from build123d import *

# Parameters (mm, degrees)
SKETCH_R        = 2.25
SKETCH_W        = 6
SKETCH_H        = 28
PAD_DEPTH       = 4.1
POCKET_DEPTH    = 3.5
SKETCH003_W     = 21
SKETCH003_H     = 4.1
POCKET001_DEPTH = 1
SKETCH002_R     = 2.25
PAD001_DEPTH    = 0.3


with BuildPart() as part:
    # Sketch → Pad (new body)
    with BuildSketch(Plane.XY):
        Polygon((-10.5, 15.5), (10.5, 15.5), (10.5, 10.499836), (6, 5.999836), (6, -5.999836), (10.5, -10.499836), (10.5, -15.5), (-10.5, -15.5), (-10.5, -17.717136), (-10.5, -19.420319), (-13.45, -19.420319), (-19.053461, -16.18516), (-19.053461, -9.71484), (-13.45, -6.479681), (-10.500002, -6.479681), (-7.46388, -3.443559), (-7.46388, 7.463716), (-10.5, 10.499836), align=None)
        with Locations((-13.45, -12.95)):
            Circle(SKETCH_R, mode=Mode.SUBTRACT)
        with Locations((0, -0.5)):
            Rectangle(SKETCH_W, SKETCH_H, mode=Mode.SUBTRACT)
    extrude(amount=PAD_DEPTH)

    # Sketch001 → Pocket (cut)
    with BuildSketch(Plane.XY.offset(4.1)):
        Polygon((-13.45, -17.020319), (-9.925, -14.98516), (-9.925, -10.91484), (-13.45, -8.879681), (-16.975, -10.91484), (-16.975, -14.98516), align=None)
    extrude(amount=-POCKET_DEPTH, mode=Mode.SUBTRACT)

    # Sketch003 → Pocket001 (cut)
    with BuildSketch(Plane(origin=(0, 15.5, 0), x_dir=(-1, 0, 0), z_dir=(0, 1, 0))):
        with Locations((0, 2.05)):
            Rectangle(SKETCH003_W, SKETCH003_H)
    extrude(amount=-POCKET001_DEPTH, mode=Mode.SUBTRACT)

    # Sketch002 → Pad001 (new body)
    with BuildSketch(Plane.XY.offset(0.6)):
        with Locations((-13.45, -12.95)):
            Circle(SKETCH002_R)
    extrude(amount=-PAD001_DEPTH)


solid = part.part
Read the model definition and answer for the solid it produces. Units are mm, in the model's axes. A direction names the side the tool comes from. Round coordinates to 2 decimals unless told otherwise and drop trailing zeros. Loops run counter-clockwise (first coordinate to the right, second up) from the corner with the lowest first, then second, coordinate; pieces in that order, holes last.
Q1. Section A-A on y = -12.95 is taken. Write down the section's boundary in (x, z) (3 decimals), and give its area (3 significant figures).
Q2. Each of these flat-tipped pins is pushed along its axis until it touches: pin 1 (1.5 mm diameter, centred on x = -11.5, z = 2.5, fed in from +Y); pin 2 (1.2 mm diameter, centred on y = 5, z = 3, fed in from +X); pin 3 (3.5 mm diameter, centred on x = -13.45, y = -12.95, fed in from +Z). Where does it stop, or does it pass through?
Q3. Which of the six approach directions +Z, -Z, +X, -X, +Y, -Y give full straight-line access (tool end or side, diameter ignored) to faces 5 (the face through (-12, -6.48, 2)), 6 (the face through (-10.5, -17, 2)), 7 (the face through (-3, -1, 2)), 8 (the face through (-16.975, -13, 2)), 9 (the face through (8, 8, 2))?
Q4. Section B-B on z = 1.75 is taken. Write down the section's boundary in (x, y) (3 decimals).
Q5. Section D-D on y = 0.5 is taken. Write down the section's boundary in (x, z), and give its area (3 significant figures).
Q6. Determine the mould class of faces 1 (the face through (-16.213, -17.825, 2.021)), 2 (the face through (-15.237, -15.988, 2.374)), 3 (the face through (-11.663, -9.912, 2.374)), 4 (the face through (10.5, 13, 2)) for opening direction X: released by +X, released by -X, zero draft, split by the parting line, or undercut.
Q7. Section C-C on x = -6.75 is taken. Write down the section's boundary in (y, z), and give its area (3 significant figures).
Q8. Consider probe 1 along X at (y, z) = (-12.5, 3.25) (3 decimals); probe 2 along X at (y, z) = (-2, 2.95); probe 3 along Y at (x, z) = (-13.45, 0.1). Determine where each line is inside the solid, lowest interval first.
Output:
1. outline: (-19.053, 0) - (-15.7, 0) - (-15.7, 0.3) - (-11.2, 0.3) - (-11.2, 0) - (-3, 0) - (-3, 4.1) - (-9.925, 4.1) - (-9.925, 0.6) - (-16.975, 0.6) - (-16.975, 4.1) - (-19.053, 4.1) - close; (3, 0) - (10.5, 0) - (10.5, 4.1) - (3, 4.1) - close
1. area: 70.5 mm2
2. pin 1: stops at y = -6.48
2. pin 2: stops at x = 6
2. pin 3: stops at z = 0.6
3. face 5: +Z, -Z, -X, +Y
3. face 6: +Z, -Z, +X, -Y
3. face 7: +Z, -Z
3. face 8: +Z
3. face 9: +Z, -Z, +X
4. outline: (-19.053, -16.185) - (-13.45, -19.42) - (-10.5, -19.42) - (-10.5, -15.5) - (10.5, -15.5) - (10.5, -10.5) - (6, -6) - (6, 6) - (10.5, 10.5) - (10.5, 14.5) - (-10.5, 14.5) - (-10.5, 10.5) - (-7.464, 7.464) - (-7.464, -3.444) - (-10.5, -6.48) - (-13.45, -6.48) - (-19.053, -9.715) - close; hole (-16.975, -14.985) - (-13.45, -17.02) - (-9.925, -14.985) - (-9.925, -10.915) - (-13.45, -8.88) - (-16.975, -10.915) - close; hole (-3, -14.5) - (3, -14.5) - (3, 13.5) - (-3, 13.5) - close
5. outline: (-7.46, 0) - (-3, 0) - (-3, 4.1) - (-7.46, 4.1) - close; (3, 0) - (6, 0) - (6, 4.1) - (3, 4.1) - close
5. area: 30.6 mm2
6. face 1: released by -X
6. face 2: undercut
6. face 3: undercut
6. face 4: released by +X
7. outline: (-15.5, 0) - (14.5, 0) - (14.5, 4.1) - (-15.5, 4.1) - close
7. area: 123 mm2
8. probe 1: x = -19.053 to -16.975, -9.925 to -3, 3 to 10.5
8. probe 2: x = -7.46 to -3, 3 to 6
8. probe 3: y = -19.42 to -15.2, -10.7 to -6.48
